Source: CAD feature listing. Evaluate the final solid. Frame: model axes, mm. A direction names the side the tool comes from. Round coordinates to 2 decimals unless told otherwise and drop trailing zeros. Loops run counter-clockwise (first coordinate to the right, second up) from the corner with the lowest first, then second, coordinate; pieces in that order, holes last.
(1) Section A-A, the plane z = 0. Return the cut outline in (x, y).
(2) Mould query, pull axis X, two halves, no side actions, for faces 1 (the flat face through (25, 6, 17.5)), 2 (the flat face through (23, 7, 0)), 3 (the cylindrical face through (24.521, 1.732, -19.595)), 4 (the cylindrical face through (26.787, 1.732, -22.498)). Classes: pulls with the +X half, pulls with the -X half, needs draft (parallel to the pull), parting line crosses it, or undercut.
(3) Set-up query: faces 5 (the flat face through (25, 6, -17.5)), 6 (the flat face through (0, 0, 0)). Return all of +Z, -Z, +X, -X, +Y, -Y with unobstructed straight access to the full face (end or side cutting, diameter ignored); none if empty.
(4) Section C-C, the plane y = 5. Return the cut outline in (x, z).
(5) First-contact query: pin 1 Ø5 at (y, z) = (8.5, 17.5) entering from -X; pin 2 Ø1.3 at (x, y) = (25, 6) entering from -Z; pin 3 Ø3 at (x, z) = (-25, -20.75) entering from -Y. Flat tips, straight axial feed; report the tip coordinate or a pass-through.
(6) Section B-B, the plane x = -20. Return the cut outline in (y, z), plus the area to 3 significant figures.
(7) Material intervals for probe 1 along X at (y, z) = (2.4, -20.75); probe 2 along X at (y, z) = (9, 12); probe 3 along Y at (x, z) = (11, 15.5), sorted ascending.
```python
from build123d import *

# Parameters (mm, degrees)
SKETCH1_R           = 1.25
BOSS_EXTRUDE1_DEPTH = 3
SKETCH2_W           = 4.5
SKETCH2_H           = 35
BOSS_EXTRUDE2_DEPTH = 8
FILLET1_R           = 1
FILLET2_R           = 2
FILLET3_R           = 0.5


with BuildPart() as part:
    # Sketch1 → Boss-Extrude1 (new body)
    with BuildSketch(Plane(origin=(0, 0, 0), x_dir=(1, 0, 0), z_dir=(0, 1, 0))):
        with BuildLine():
            Line((-27.5, -19.25), (-27.5, -20.75))
            ThreePointArc((-27.5, -20.75), (-26.767766953, -22.517766953), (-25, -23.25))
            Line((-25, -23.25), (25, -23.25))
            ThreePointArc((25, -23.25), (26.767766953, -22.517766953), (27.5, -20.75))
            Line((27.5, -20.75), (27.5, 20.75))
            ThreePointArc((27.5, 20.75), (26.767766953, 22.517766953), (25, 23.25))
            Line((25, 23.25), (-25, 23.25))
            ThreePointArc((-25, 23.25), (-26.767766953, 22.517766953), (-27.5, 20.75))
            Line((-27.5, 20.75), (-27.5, 19.25))
            Line((-27.5, 19.25), (-27.5, -19.25))
        make_face()
        with Locations(Location((-25, -20.75, 0), (0, 0, 270))):
            Circle(SKETCH1_R, mode=Mode.SUBTRACT)
        with Locations(Location((25, -20.75, 0), (0, 0, 270))):
            Circle(SKETCH1_R, mode=Mode.SUBTRACT)
        with Locations(Location((25, 20.75, 0), (0, 0, 270))):
            Circle(SKETCH1_R, mode=Mode.SUBTRACT)
        with Locations(Location((-25, 20.75, 0), (0, 0, 270))):
            Circle(SKETCH1_R, mode=Mode.SUBTRACT)
    extrude(amount=BOSS_EXTRUDE1_DEPTH)

    # Sketch2 → Boss-Extrude2 (add)
    with BuildSketch(Plane(origin=(0, 3, 0), x_dir=(1, 0, 0), z_dir=(0, 1, 0))):
        with Locations((25.25, 0)):
            Rectangle(SKETCH2_W, SKETCH2_H)
    extrude(amount=BOSS_EXTRUDE2_DEPTH)

    # Fillet1
    fillet1_edges = [part.edges().sort_by_distance(p)[0] for p in [
        (25.25, 3, -17.5),
        (25.25, 3, 17.5),
    ]]
    fillet(fillet1_edges, radius=FILLET1_R)

    # Fillet2
    fillet2_edges = [part.edges().sort_by_distance(p)[0] for p in [
        (25.25, 11, -17.5),
        (25.25, 11, 17.5),
    ]]
    fillet(fillet2_edges, radius=FILLET2_R)

    # Fillet3
    fillet3_edges = [part.edges().sort_by_distance(p)[0] for p in [
        (-27.5, 0, 0),
        (-26.767766953, 0, -22.517766953),
        (0, 0, -23.25),
        (26.767766953, 0, -22.517766953),
        (27.5, 0, 0),
        (26.767766953, 0, 22.517766953),
        (0, 0, 23.25),
        (-26.767766953, 0, 22.517766953),
        (-25, 0, 19.5),
        (25, 0, 19.5),
        (25, 0, -22),
        (-25, 0, -22),
    ]]
    fillet(fillet3_edges, radius=FILLET3_R)


solid = part.part
```
Output values:
1. outline: (-27.5, 0.5) arc R0.5 ccw to (-27, 0) - (27, 0) arc R0.5 ccw to (27.5, 0.5) - (27.5, 11) - (23, 11) - (23, 3) - (-27.5, 3) - close
2. face 1: needs draft
2. face 2: pulls with the -X half
2. face 3: undercut
2. face 4: pulls with the +X half
3. face 5: -Z, +X, -X, +Y
3. face 6: +Z, -Z, +X, -X, -Y
4. outline: (23, -17.5) - (27.5, -17.5) - (27.5, 17.5) - (23, 17.5) - close
5. pin 1: stops at x = 23
5. pin 2: stops at z = -17.5
5. pin 3: stops at y = 0.07
6. outline: (0, -22.75) arc R0.5 ccw to (0.5, -23.25) - (3, -23.25) - (3, 23.25) - (0.5, 23.25) arc R0.5 ccw to (0, 22.75) - close
6. area: 139 mm2
7. probe 1: x = -27.5 to -26.25, -23.75 to 23.75, 26.25 to 27.5
7. probe 2: x = 23 to 27.5
7. probe 3: y = 0 to 3
